```python
from build123d import *

# Parameters (mm, degrees)
F0_W     = 834.740075
F0_H     = 50.8
F1_DEPTH = 5.08
F3_W     = 57.9247
F3_H     = 5.334
F3_W_2   = 115.8494
F4_DEPTH = 5.08
F5_W     = 5.334
F5_H     = 30.48
F6_DEPTH = 25.4
F7_R     = 1.27
F8_DEPTH = 5.081


with BuildPart() as f1:
    # F0 (on Front) → F1 (new body)
    with BuildSketch(Plane.XZ):
        with Locations((417.370037, 25.4)):
            Rectangle(F0_W, F0_H)
    extrude(amount=F1_DEPTH)

    # F3 (on face) → F4 (join)
    with BuildSketch(Plane.XZ.offset(5.08)):
        with Locations((28.96235, 53.467)):
            Rectangle(F3_W, F3_H)
        with Locations((139.123346, 53.467)):
            Rectangle(F3_W_2, F3_H)
        with Locations((28.96235, -2.667)):
            Rectangle(F3_W, F3_H)
        with Locations((139.123346, -2.667)):
            Rectangle(F3_W_2, F3_H)
        with Locations((278.246692, 53.467)):
            Rectangle(F3_W_2, F3_H)
        with Locations((278.246692, -2.667)):
            Rectangle(F3_W_2, F3_H)
        with Locations((417.370038, 53.467)):
            Rectangle(F3_W_2, F3_H)
        with Locations((417.370038, -2.667)):
            Rectangle(F3_W_2, F3_H)
        with Locations((556.493384, 53.467)):
            Rectangle(F3_W_2, F3_H)
        with Locations((556.493384, -2.667)):
            Rectangle(F3_W_2, F3_H)
        with Locations((695.61673, 53.467)):
            Rectangle(F3_W_2, F3_H)
        with Locations((695.61673, -2.667)):
            Rectangle(F3_W_2, F3_H)
        with Locations((805.777725, 53.467)):
            Rectangle(F3_W, F3_H)
        with Locations((805.777725, -2.667)):
            Rectangle(F3_W, F3_H)
    extrude(amount=-F4_DEPTH)

    # F5 (on face) → F6 (cut)
    with BuildSketch(Plane(origin=(0, 0, 0), x_dir=(-1, 0, 0), z_dir=(0, 1, 0))):
        with Locations((-646.70903, 9.906)):
            Rectangle(F5_W, F5_H)
        with Locations((-48.9077, 9.906)):
            Rectangle(F5_W, F5_H)
    extrude(amount=-F6_DEPTH, mode=Mode.SUBTRACT)

    # F7 (on face) → F8 (cut, through all)
    with BuildSketch(Plane(origin=(0, 0, 0), x_dir=(-1, 0, 0), z_dir=(0, 1, 0))):
        with Locations((-695.61673, 25.4)):
            Circle(F7_R)
        with Locations((-695.61673, 31.75)):
            Circle(F7_R)
        with Locations((-828.390075, 31.75)):
            Circle(F7_R)
        with Locations((-828.390075, 25.4)):
            Circle(F7_R)
    extrude(amount=-F8_DEPTH, mode=Mode.SUBTRACT)


solid = f1.part
```
Work out the finished part from the listing and answer in its coordinate system (mm). Round coordinates to 2 decimals unless told otherwise and drop trailing zeros.
1) A cutting plane is placed at A-A on y = -1.8. Give the number of separate pieces and of enclosed holes in the cut face, and give its area (3 significant figures).
2) A flat-ended cylindrical pin translates along its axis: P1, Ø1.5, axis at x = 760.5, y = -2.5, coming from the +Z side. Find the tip coordinate at first contact, or state that the pin passes through.
3) Consider probe 1 along X at (y, z) = (-4.3, 32); probe 2 along X at (y, z) = (-4.65, 12); probe 3 along Z at (x, y) = (68.5, -2.1). Determine where each line is inside the solid, lowest interval first.
Entries:
1. separate pieces: 1
1. enclosed holes: 4
1. area: 49,500 mm2
2. P1: stops at z = 50.8
3. probe 1: x = 0 to 694.37, 696.86 to 827.14, 829.64 to 834.74
3. probe 2: x = 0 to 46.24, 51.57 to 644.04, 649.38 to 834.74
3. probe 3: z = 0 to 50.8
